```python
from build123d import *

# Parameters (mm, degrees)
CROQUIS1_R              = 11
CROQUIS1_R_2            = 4
SALIENTE_EXTRUIR1_DEPTH = 2
CROQUIS2_R              = 5
CROQUIS2_R_2            = 3
SALIENTE_EXTRUIR2_DEPTH = 10
CROQUIS3_R              = 1.75
CORTAR_EXTRUIR1_DEPTH   = 10


with BuildPart() as part:
    # Croquis1 → Saliente-Extruir1 (new body)
    with BuildSketch(Plane(origin=(0, 0, 0), x_dir=(1, 0, 0), z_dir=(0, 1, 0))):
        with Locations(Location((0, 0, 0), (0, 0, 270))):
            Circle(CROQUIS1_R)
        with Locations(Location((0, 0, 0), (0, 0, 270))):
            Circle(CROQUIS1_R_2, mode=Mode.SUBTRACT)
    extrude(amount=SALIENTE_EXTRUIR1_DEPTH)

    # Croquis2 → Saliente-Extruir2 (add)
    with BuildSketch(Plane(origin=(0, 2, 0), x_dir=(1, 0, 0), z_dir=(0, 1, 0))):
        with Locations(Location((0, 0, 0), (0, 0, 270))):
            Circle(CROQUIS2_R)
        with Locations(Location((0, 0, 0), (0, 0, 270))):
            Circle(CROQUIS2_R_2, mode=Mode.SUBTRACT)
    extrude(amount=SALIENTE_EXTRUIR2_DEPTH)

    # Croquis3 → Cortar-Extruir1 (cut)
    with BuildSketch(Plane.XZ):
        with Locations(Location((0, 8, 0), (0, 0, 270))):
            Circle(CROQUIS3_R)
        with Locations(Location((8, 0, 0), (0, 0, 270))):
            Circle(CROQUIS3_R)
        with Locations(Location((-8, 0, 0), (0, 0, 270))):
            Circle(CROQUIS3_R)
        with Locations(Location((0, -8, 0), (0, 0, 270))):
            Circle(CROQUIS3_R)
    extrude(amount=-CORTAR_EXTRUIR1_DEPTH, mode=Mode.SUBTRACT)


solid = part.part
```
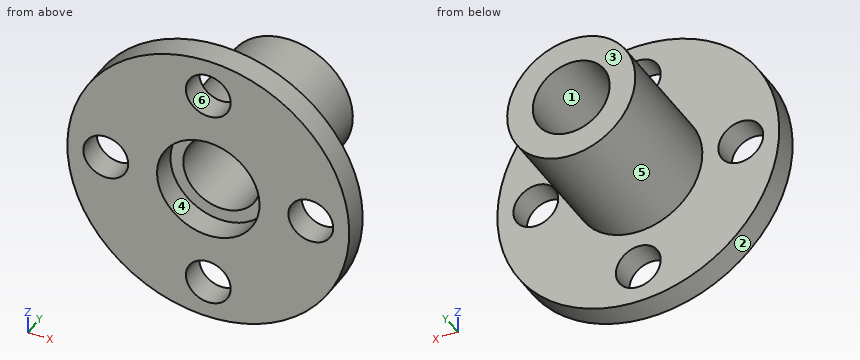
CAD build for the part. Positions are in the model's coordinates, mm. Face numbers are marked on the shaded views. A direction names the side the tool comes from. Give positions to 0.01 mm unless a question says otherwise; leave off trailing zeros. Loops run counter-clockwise (first coordinate to the right, second up) from the corner with the lowest first, then second, coordinate; pieces in that order, holes last. Notation, with made-up numbers: (-8, 58.25) -> (10, 58.25) arc R12 ccw to (10, 73.25) -> close; hole circle Ø11 at (-19, -26). An arc over 180 degrees is marked (long way). Use a Markdown table: item, result.
1. Wall check: L1, parallel to X at y = 1.25, z = 0; L2, parallel to Y at x = 9.5, z = 3.25; L3, parallel to Z at x = 1.5, y = 9. Give the ranges that are in metal, low to high. Write a range as [from, to].
Check result:
| item | result |
|---|---|
| L1 | x = [-11, -9.75], [-6.25, -4], [4, 6.25], [9.75, 11] |
| L2 | y = [0, 2] |
| L3 | z = [-4.77, -2.6], [2.6, 4.77] |
2. Flat gauge pins, fed straight in: pin 1 (6 mm diameter, centred on x = -3, z = 7.5, fed in from +Y); pin 2 (2 mm diameter, centred on x = 0, z = -8, fed in from +Y); pin 3 (4 mm diameter, centred on x = -1, z = 1.5, fed in from -Y); pin 4 (5 mm diameter, centred on y = 3, z = -8.5, fed in from +X). Where does each tip first touch, or does it go through?
Check result:
| item | result |
|---|---|
| pin 1 | stops at y = 2 |
| pin 2 | passes through |
| pin 3 | stops at y = 2 |
| pin 4 | stops at x = 9.08 |
3. Mould opens along Z. For the marked faces 1, 2 and 3 say: pulls with the +Z half, pulls with the -Z half, needs draft (parallel to the pull), parting line crosses it, or undercut.
Check result:
| item | result |
|---|---|
| face 1 | undercut |
| face 2 | parting line crosses it |
| face 3 | needs draft |
4. Slice it at A-A (z = -8.75). List the corners of the cut face in (x, y).
Check result:
| item | result |
|---|---|
| outline | (-6.67, 0) -> (-1.58, 0) -> (-1.58, 2) -> (-6.67, 2) -> close; (1.58, 0) -> (6.67, 0) -> (6.67, 2) -> (1.58, 2) -> close |
5. Slice it at C-C (y = 9.75). List the corners of the cut face in (x, z).
Check result:
| item | result |
|---|---|
| outline | circle Ø10 at (0, 0); hole circle Ø6 at (0, 0) |
6. Slice it at B-B (x = 8). List the corners of the cut face in (y, z).
Check result:
| item | result |
|---|---|
| outline | (0, -7.55) -> (2, -7.55) -> (2, -1.75) -> (0, -1.75) -> close; (0, 1.75) -> (2, 1.75) -> (2, 7.55) -> (0, 7.55) -> close |
7. Which spindle directions (+Z, -Z, +X, -X, +Y, -Y) get a long thin tool onto all of the face, cutting with end or side? Do the marked faces 4, 5 and 6. Say none if no direction does.
Check result:
| item | result |
|---|---|
| face 4 | -Y |
| face 5 | +Y |
| face 6 | +Y, -Y |
8. Slice it at D-D (x = -1.25). List the corners of the cut face in (y, z), plus the area to 3 significant figures.
Check result:
| item | result |
|---|---|
| outline | (0, -10.93) -> (2, -10.93) -> (2, -9.22) -> (0, -9.22) -> close; (0, -6.78) -> (2, -6.78) -> (2, -4.84) -> (12, -4.84) -> (12, -2.73) -> (2, -2.73) -> (2, -3.8) -> (0, -3.8) -> close; (0, 3.8) -> (2, 3.8) -> (2, 2.73) -> (12, 2.73) -> (12, 4.84) -> (2, 4.84) -> (2, 6.78) -> (0, 6.78) -> close; (0, 9.22) -> (2, 9.22) -> (2, 10.93) -> (0, 10.93) -> close |
| area | 61.0 mm^2 |
